Autodesk Inventor part; units mm, degrees
ref_plane "MSC_PF1" through (0, 0, 0) normal (1, 0, 0) x (0, 1, 0)
ref_plane "MSC_PT1" through (0, 0, 0) normal (0, 0, -1) x (-1, 0, 0)
ref_plane "YZ Plane" through (0, 0, 0) normal (1, 0, 0) x (0, 1, 0)
sketch "Esquisse1" plane through (0, 0, 0) normal (0, 1, 0) x (-1, 0, 0)
  point P0 (0, 0)
sketch "Esquisse2" plane through (0, 0, 0) normal (0, 0, 1) x (1, 0, 0)
  point P0 (0, 0)
sketch "Esquisse3" plane through (0, 0, 0) normal (0, 0, 1) x (1, 0, 0)
  point P0 (0, 0)
sketch "Esquisse4" plane through (0, 0, 0) normal (0, 1, 0) x (-1, 0, 0)
  line L0 (-2.75, 0) -> (0, 0)
  line L1 (-2.75, -0.4) -> (-2.75, 0)
  line L2 (-1.5, -1.65) -> (-2.75, -0.4)
  line L3 (-1.5, -1.9) -> (-1.5, -1.65)
  line L4 (-1.25, -2.15) -> (-1.5, -1.9)
  line L5 (-1.5, -2.4) -> (-1.25, -2.15)
  line L6 (-1.5, -12) -> (-1.5, -2.4)
  line L7 (0, 0) -> (0, -12)
  line L8 (0, 3.3392) -> (0, -10.7) construction
  line L9 (0, 3.3392) -> (0, -10.7)
  line L10 (0, -15.0678) -> (0, 6.4071)
  line L11 (-1.5, -12) -> (0, -12)
  line L12 (0.55, 0) -> (-3.3, 0)
  dimension "d3" = 2.75
  dimension "d5" = 0.25
  dimension "d7" = 0.25
  dimension "d9" = 0.25
  dimension "d11" = 1.65
  dimension "d13" = 135
  dimension "d17" = 1.25
  dimension "d19" = 0
  dimension "d51" = 1.5
  dimension "d52" = 12
revolve "Révolution1" add sketch "Esquisse4" angle 360 about axis through (0, 0, 3.3392) along (0, 0, -1)
sketch "Esquisse5" plane through (0, 0, 0) normal (0, 1, 0) x (-1, 0, 0)
  line L0 (-1.6, 0) -> (0, 0)
  line L1 (-0.2667, -1.5) -> (-1.6, 0)
  line L2 (0, -1.5) -> (-0.2667, -1.5)
  line L3 (0, 0) -> (0, -1.5)
  line L4 (-1.5, -1.65) -> (1.5, -1.65) construction
  line L5 (-2.75, 0) -> (2.75, 0)
  line L6 (0, -1.98) -> (0, 0.33)
  dimension "d22" = 1.6
  dimension "d24" = 0.2667
  dimension "d26" = 1.5
extrude "Extrusion1" cut sketch "Esquisse5" along normal mid plane 0.5333
pattern_circular "RéseauPolaire1" count 4 over 360 about axis through (0, 0, 0) along (0, 0, 1) of "Extrusion1"
sketch "Esquisse7" plane through (0, 0, 0) normal (0, 1, 0) x (-1, 0, 0)
  line L0 (0, -0.825) -> (-2, 0)
  line L1 (0, 0) -> (0, -0.825)
  line L2 (-2, 0) -> (0, 0)
  line L3 (-1.5, -1.65) -> (1.5, -1.65) construction
  line L4 (0, -1.98) -> (0, 0.33)
  line L5 (-2.75, 0) -> (2.75, 0)
  dimension "d33" = 2
  dimension "d35" = 0.825
extrude "Extrusion2" cut sketch "Esquisse7" along normal mid plane 0.5333
pattern_circular "RéseauPolaire2" count 4 over 360 about axis through (0, 0, 0) along (0, 0, 1) of "Extrusion2"
fillet "Congé1" radius 0.5 1 edges at (-1.5, 0, -1.65)
thread "Filetage1"
ref_plane "MSC_PF1" through (0, 0, 0) normal (1, 0, 0) x (0, 1, 0)
ref_plane "MSC_PT1" through (0, 0, 0) normal (0, 0, -1) x (-1, 0, 0)
equation "\"d3\" = 0.5 * Dh"
equation "\"d5\" = msp_x"
equation "\"d7\" = ParA"
equation "\"d9\" = msp_x"
equation "\"d11\" = ParK"
equation "\"d17\" = 0.5 * msp_mdtds"
equation "\"d51\" = 0.5 * NND"
equation "\"d52\" = NLG"
equation "\"d22\" = 0.5 * M"
equation "\"d24\" = 0.0833333 * M"
equation "\"d26\" = 0.909091 * ParK"
equation "\"d27\" = 0.166667 * M"
equation "\"d33\" = 0.625 * M"
equation "\"d35\" = 0.5 * ParK"
equation "\"d36\" = 0.166667 * M"
equation "\"d41\" = 2 * msp_x"
equation "\"PTC\" = 0.5"
equation "\"NLG\" = 12"
equation "\"ParK\" = 1.65"
equation "\"NND\" = 3"
equation "\"M\" = 3.2"
equation "\"msp_mdtds\" = NND - PTC"
equation "\"Dh\" = 5.5"
equation "\"msp_x\" = 0.5 * PTC"
equation "\"ParA\" = 0.5 * PTC"
equation "\"r\" = 0.8"
equation "\"THREADDIA\" = NND"
equation "\"TEMPLATE\" = 1.2345"
properties part number "NF EN ISO 7046-2 H - M3x12 - 8.8 - H1" material "Acier inoxydable 440C"
The listing builds one solid part. Answer for the finished solid, in the listing's coordinates (mm). A direction names the side the tool comes from. Round coordinates to 2 decimals unless told otherwise and drop trailing zeros. Order: outer loops, then holes, each group sorted by start corner. A loop starts at its lowest first (then second) coordinate and runs counter-clockwise, first axis right, second up. Notation, with made-up numbers: (83, 86) -> (110, 86) arc R33 cw to (110, 115) -> close; hole circle Ø9 at (-8, -17). An arc over 180 degrees is marked (long way). Answer as CSV lines item,"result".
Q1. Given pin 1 (0.8 mm diameter, centred on x = -1, z = -1, fed in from +Y); pin 2 (1.5 mm diameter, centred on x = -1.5, z = -10.5, fed in from +Y); pin 3 (0.5 mm diameter, centred on y = 1.5, z = -1, fed in from -X), each flat-ended and moving along its own axis, determine where each tip first touches the part or whether it passes through.
Computed values:
pin 1,"stops at y = 2.37"
pin 2,"stops at y = 1.3"
pin 3,"stops at x = -1.93"
Q2. Consider line 1 (Y direction, x = -0.1, z = -9.25); line 2 (X direction, y = -1.2, z = -1). Determine where each line is inside the solid, lowest interval first. Write a range as from..to.
Computed values:
line 1,"y = -1.5..1.5"
line 2,"x = -1.78..1.78"
Q3. For a pull along X with two mould halves and no side action, classify faces 1 (the cylindrical face through (-1.5, 0.07, -7.13)), 2 (the flat face through (0.8, 0, -0.9)), 3 (the flat face through (1, 1, 0)) as +X half, -X half, draft (parallel to the pull), parting line (faces both ways), or undercut.
Computed values:
face 1,"parting line"
face 2,"undercut"
face 3,"draft"
Q4. A cutting plane is placed at A-A on z = -7.5. Determine the outline of the cut face in (x, y), plus the area to 3 significant figures.
Computed values:
outline,"circle Ø3 at (0, 0)"
area,"7.07 mm^2"
Q5. Which of the six approach directions +Z, -Z, +X, -X, +Y, -Y give full straight-line access (tool end or side, diameter ignored) to faces 4 (the flat face through (0.8, 0.267, -0.4)), 5 (the cylindrical face through (-0.596, -2.685, -0.197))?
Computed values:
face 4,"+Z"
face 5,"+Z, -Z"
